Verification items for the finished model (mm, model axes). Coordinates: 2 decimals unless noted, no trailing zeros. Loops run counter-clockwise (first coordinate to the right, second up) from the corner with the lowest first, then second, coordinate; pieces in that order, holes last. Notation, with made-up numbers: (-6.5, -20.5) -> (25.5, -20.5) arc R20 cw to (25.5, 13.5) -> close; hole circle Ø9 at (-4, 63.25). An arc over 180 degrees is marked (long way). Write item = value, one per line.
```python
from build123d import *

# Parameters (mm, degrees)
SKETCH1_R           = 2.5
SKETCH1_R_2         = 6
BOSS_EXTRUDE1_DEPTH = 7
FILLET1_R           = 5
FILLET2_R           = 1


with BuildPart() as part:
    # Sketch1 → Boss-Extrude1 (new body)
    # profile 1 of 2: a face of its own
    with BuildSketch(Plane.XY):
        with BuildLine():
            Line((-5.942775796, 0.826689684), (-17.7, -83.691780519))
            Line((-17.7, -83.691780519), (-17.7, -106.6))
            Line((-17.7, -106.6), (68.5, -106.6))
            Line((68.5, -106.6), (68.5, -83.691780519))
            Line((68.5, -83.691780519), (4.84674687, 3.5368128))
            ThreePointArc((4.84674687, 3.5368128), (5.704405369, 1.860042846), (6, 0))
            ThreePointArc((6, 0), (-0.414333936, -5.985676853), (-5.942775796, 0.826689684))
        make_face()
        with Locations((-12.7, -101.6)):
            Circle(SKETCH1_R, mode=Mode.SUBTRACT)
        with Locations((-12.7, -88.9)):
            Circle(SKETCH1_R, mode=Mode.SUBTRACT)
        with Locations((63.5, -101.6)):
            Circle(SKETCH1_R, mode=Mode.SUBTRACT)
        with Locations((63.5, -88.9)):
            Circle(SKETCH1_R, mode=Mode.SUBTRACT)
    # profile 2 of 2: a face of its own
    with BuildSketch(Plane.XY):
        Circle(SKETCH1_R_2)
        Circle(SKETCH1_R, mode=Mode.SUBTRACT)
    extrude(amount=BOSS_EXTRUDE1_DEPTH)

    # Fillet1
    fillet1_edges = [part.edges().sort_by_distance(p)[0] for p in [
        (68.5, -83.691780519, 3.5),
        (68.5, -106.6, 3.5),
        (-17.7, -106.6, 3.5),
        (-17.7, -83.691780519, 3.5),
    ]]
    fillet(fillet1_edges, radius=FILLET1_R)

    # Fillet2
    fillet2_edges = [part.edges().sort_by_distance(p)[0] for p in [
        (-1.461681114, 5.819234342, 7),
        (-1.461681114, 5.819234342, 0),
        (-17.7, -92.818942509, 0),
        (-17.7, -92.818942509, 7),
        (36.192851297, -39.418990098, 0),
        (68.5, -93.461068497, 0),
        (25.4, -106.6, 0),
        (-11.79754448, -41.261143632, 0),
        (-16.235533906, -105.135533906, 0),
        (67.035533906, -105.135533906, 0),
        (68.25367114, -83.77210129, 0),
        (-17.688064044, -83.692606737, 0),
        (-11.79754448, -41.261143632, 7),
        (36.192851297, -39.418990098, 7),
        (25.4, -106.6, 7),
        (68.5, -93.461068497, 7),
        (-16.235533906, -105.135533906, 7),
        (67.035533906, -105.135533906, 7),
        (68.25367114, -83.77210129, 7),
        (-17.688064044, -83.692606737, 7),
    ]]
    fillet(fillet2_edges, radius=FILLET2_R)


solid = part.part
```
1) Depth check by flat-ended pin: pin 1 Ø10 at (x, y) = (4, -83) entering from -Z; pin 2 Ø1 at (y, z) = (-77, 3.5) entering from -X; pin 3 Ø4 at (y, z) = (-23.5, 2) entering from -X. Enter the tip coordinate at first touch or a pass-through.
Ans:
pin_1 = 0
pin_2 = -16.84
pin_3 = -9.61
2) Sectioned sample at B-B, the plane z = 3. Record the cut outline in (x, y).
Ans:
outline = (-17.7, -101.6) arc R5 ccw to (-12.7, -106.6) -> (63.5, -106.6) arc R5 ccw to (68.5, -101.6) -> (68.5, -85.32) arc R5 ccw to (67.54, -82.37) -> (4.85, 3.54) arc R6 ccw to (-5.94, 0.83) -> (-17.65, -83.35) arc R5 ccw to (-17.7, -84.04) -> close; hole circle Ø5 at (-12.7, -101.6); hole circle Ø5 at (-12.7, -88.9); hole circle Ø5 at (0, 0); hole circle Ø5 at (63.5, -101.6); hole circle Ø5 at (63.5, -88.9)
3) Release check for a two-part mould opening along X. For faces 1 (the face through (36.63, -40.02, 3.46)), 2 (the face through (-1.365, 5.843, 3.465)), 3 (the face through (15, -62, 0)), 4 (the face through (63.17, -86.42, 3.45)) record: pulls with the +X half, pulls with the -X half, needs draft (parallel to the pull), parting line crosses it, or undercut.
Ans:
face_1 = pulls with the +X half
face_2 = parting line crosses it
face_3 = needs draft
face_4 = undercut
4) Sectioned sample at A-A, the plane y = -88.9. Record the cut outline in (x, z), plus the area to 3 significant figures.
Ans:
outline = (-17.7, 1) arc R1 ccw to (-16.7, 0) -> (-15.2, 0) -> (-15.2, 7) -> (-16.7, 7) arc R1 ccw to (-17.7, 6) -> close; (-10.2, 0) -> (61, 0) -> (61, 7) -> (-10.2, 7) -> close; (66, 0) -> (67.5, 0) arc R1 ccw to (68.5, 1) -> (68.5, 6) arc R1 ccw to (67.5, 7) -> (66, 7) -> close
area = 533 mm2
5) Material ranges on line 1 (Y direction, x = 0, z = 2); line 2 (Y direction, x = 63.5, z = 3); line 3 (Y direction, x = 14, z = 2.75), recorded low to high.
Ans:
line_1 = -106.6 to -2.5, 2.5 to 6
line_2 = -106.6 to -104.1, -99.1 to -91.4, -86.4 to -76.84
line_3 = -106.6 to -9.01
